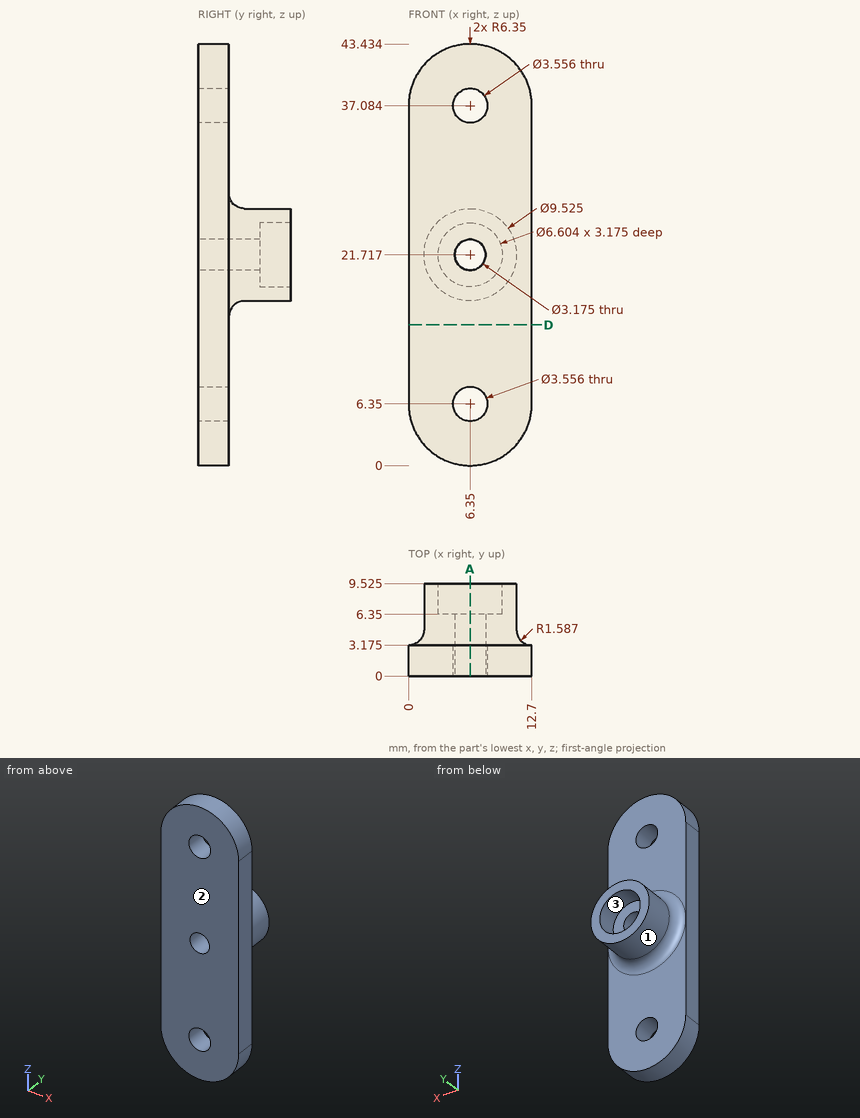
Source: three-view drawing plus pictorial views. Frame: mm from the lowest corner of the part. Round coordinates to 2 decimals unless told otherwise and drop trailing zeros. Order: outer loops, then holes, each group sorted by start corner. A loop starts at its lowest first (then second) coordinate and runs counter-clockwise, first axis right, second up. Notation, with made-up numbers: (74, 73.25) - (90, 73.25) arc R31 ccw to (90, 110.25) - close; hole circle Ø6 at (-3.75, 30.5). An arc over 180 degrees is marked (long way). Use a Markdown table: item, result.
1. Section D-D on z = 14.5. Return the cut outline in (x, y) (1 decimal).
Evaluation:
| item | result |
|---|---|
| outline | (0, 0) - (12.7, 0) - (12.7, 3.2) - (0, 3.2) - close |
2. First-contact query: pin 1 (4.5 mm diameter, centred on x = 6.35, z = 37.084, fed in from +Y) (3 decimals); pin 2 (1 mm diameter, centred on x = 2, y = 1, fed in from -Z); pin 3 (4 mm diameter, centred on x = 8.5, y = 1.5, fed in from +Z). Flat tips, straight axial feed; report the tip coordinate or a pass-through.
Evaluation:
| item | result |
|---|---|
| pin 1 | y = 3.175 |
| pin 2 | z = 1.3 |
| pin 3 | z = 43.43 |
3. Section A-A on x = 6.35. State how many separate pieces and enclosed holes the cut face has, then the cut area to 3 significant figures.
Evaluation:
| item | result |
|---|---|
| separate pieces | 4 |
| enclosed holes | 0 |
| area | 136 mm^2 |
4. Mould query, pull axis X, two halves, no side actions, for the marked faces 1, 2 and 3. Classes: +X half, -X half, draft (parallel to the pull), parting line (faces both ways), or undercut.
Evaluation:
| item | result |
|---|---|
| face 1 | parting line |
| face 2 | draft |
| face 3 | undercut |
5. Material intervals for probe 1 along X at (y, z) = (1.25, 6.5); probe 2 along Y at (x, z) = (9.25, 32.5) (1 decimal); probe 3 along Y at (x, z) = (7.25, 24.5), sorted ascending.
Evaluation:
| item | result |
|---|---|
| probe 1 | 0 to 4.58, 8.12 to 12.7 |
| probe 2 | 0 to 3.2 |
| probe 3 | 0 to 6.35 |
